Input: part model. Units: mm. Frame: model coordinates. Round coordinates to 2 decimals unless told otherwise and drop trailing zeros. Loops run counter-clockwise (first coordinate to the right, second up) from the corner with the lowest first, then second, coordinate; pieces in that order, holes last. Notation, with made-up numbers: M -14,-33 L 43,-33 A17 ccw 43,-7 Z; hole C 4,71.5 d2. An arc over 180 degrees is marked long. Put each result on its own line as item: value. Start each with the question number.
1) Section A-A on x = 116. Output: boundary loops of the cut face in (y, z).
2) Section C-C on y = 0.95. State how many separate pieces and enclosed holes the cut face has, plus the area to 3 significant figures.
3) Section B-B on z = -50. Output: boundary loops of the cut face in (x, y), plus the area to 3 significant figures.
4) Line query: probe 1 along X at (y, z) = (0.45, -28); probe 2 along Z at (x, y) = (97.5, 0.8); probe 3 along X at (y, z) = (0.7, -50). Output: solid intervals per line, ascending.
5) Pin query (flat end, axial travel): pin 1 (6 mm diameter, centred on x = 27.5, z = -31.5, fed in from +Y). Return the tip coordinate at first contact, or that it passes through.
6) Section D-D on z = -28. Output: boundary loops of the cut face in (x, y).
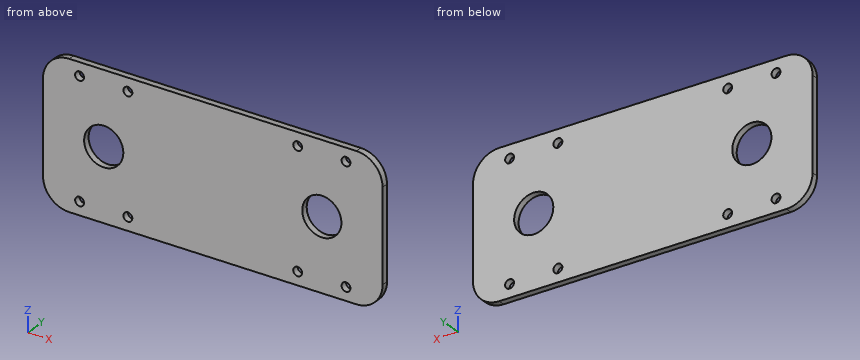
from build123d import *

# Parameters (mm, degrees)
BOSS_EXTRUDE1_DEPTH = 2.5
SKETCH2_R           = 1.7
CUT_EXTRUDE1_DEPTH  = 142.178079035
SKETCH3_R           = 1.7
CUT_EXTRUDE2_DEPTH  = 10
SKETCH4_R           = 7.5
CUT_EXTRUDE3_DEPTH  = 10


with BuildPart() as part:
    # Sketch1 → Boss-Extrude1 (new body)
    with BuildSketch(Plane(origin=(0, 0, 0), x_dir=(1, 0, 0), z_dir=(0, 1, 0))):
        with BuildLine():
            Line((10, 0), (120, 0))
            ThreePointArc((120, 0), (127.071067812, 2.928932188), (130, 10))
            Line((130, 10), (130, 45))
            ThreePointArc((130, 45), (127.071067812, 52.071067812), (120, 55))
            Line((120, 55), (10, 55))
            ThreePointArc((10, 55), (2.928932188, 52.071067812), (0, 45))
            Line((0, 45), (0, 10))
            ThreePointArc((0, 10), (2.928932188, 2.928932188), (10, 0))
        make_face()
    extrude(amount=BOSS_EXTRUDE1_DEPTH)

    # Sketch2 → Cut-Extrude1 (cut, through all)
    with BuildSketch(Plane(origin=(0, 2.5, 0), x_dir=(1, 0, 0), z_dir=(0, 1, 0))):
        with Locations(Location((14, 5, 0), (0, 0, 270))):
            Circle(SKETCH2_R)
        with Locations(Location((14, 50, 0), (0, 0, 270))):
            Circle(SKETCH2_R)
        with Locations(Location((116, 5, 0), (0, 0, 90))):
            Circle(SKETCH2_R)
        with Locations(Location((116, 50, 0), (0, 0, 90))):
            Circle(SKETCH2_R)
    extrude(amount=-CUT_EXTRUDE1_DEPTH, mode=Mode.SUBTRACT)

    # Sketch3 → Cut-Extrude2 (cut)
    with BuildSketch(Plane(origin=(0, 2.5, 0), x_dir=(1, 0, 0), z_dir=(0, 1, 0))):
        with Locations(Location((32.5, 50, 0), (0, 0, 270))):
            Circle(SKETCH3_R)
        with Locations(Location((32.5, 5, 0), (0, 0, 270))):
            Circle(SKETCH3_R)
        with Locations(Location((97.5, 5, 0), (0, 0, 270))):
            Circle(SKETCH3_R)
        with Locations(Location((97.5, 50, 0), (0, 0, 270))):
            Circle(SKETCH3_R)
    extrude(amount=-CUT_EXTRUDE2_DEPTH, mode=Mode.SUBTRACT)

    # Sketch4 → Cut-Extrude3 (cut)
    with BuildSketch(Plane(origin=(0, 2.5, 0), x_dir=(1, 0, 0), z_dir=(0, 1, 0))):
        with Locations(Location((23.25, 27.5, 0), (0, 0, 270))):
            Circle(SKETCH4_R)
        with Locations(Location((106.75, 27.5, 0), (0, 0, 270))):
            Circle(SKETCH4_R)
    extrude(amount=-CUT_EXTRUDE3_DEPTH, mode=Mode.SUBTRACT)


solid = part.part
Geometry results:
1. outline: M 0,-55 L 2.5,-55 L 2.5,-51.7 L 0,-51.7 Z; M 0,-48.3 L 2.5,-48.3 L 2.5,-6.7 L 0,-6.7 Z; M 0,-3.3 L 2.5,-3.3 L 2.5,0 L 0,0 Z
2. separate pieces: 1
2. enclosed holes: 10
2. area: 6,640 mm²
3. outline: M 1.34,0 L 12.3,0 L 12.3,2.5 L 1.34,2.5 Z; M 15.7,0 L 30.8,0 L 30.8,2.5 L 15.7,2.5 Z; M 34.2,0 L 95.8,0 L 95.8,2.5 L 34.2,2.5 Z; M 99.2,0 L 114.3,0 L 114.3,2.5 L 99.2,2.5 Z; M 117.7,0 L 128.66,0 L 128.66,2.5 L 117.7,2.5 Z
3. area: 284 mm²
4. probe 1: x = 0 to 15.77, 30.73 to 99.27, 114.23 to 130
4. probe 2: z = -55 to -51.7, -48.3 to -6.7, -3.3 to 0
4. probe 3: x = 1.34 to 12.3, 15.7 to 30.8, 34.2 to 95.8, 99.2 to 114.3, 117.7 to 128.66
5. pin 1: stops at y = 2.5
6. outline: M 0,0 L 15.77,0 L 15.77,2.5 L 0,2.5 Z; M 30.73,0 L 99.27,0 L 99.27,2.5 L 30.73,2.5 Z; M 114.23,0 L 130,0 L 130,2.5 L 114.23,2.5 Z
